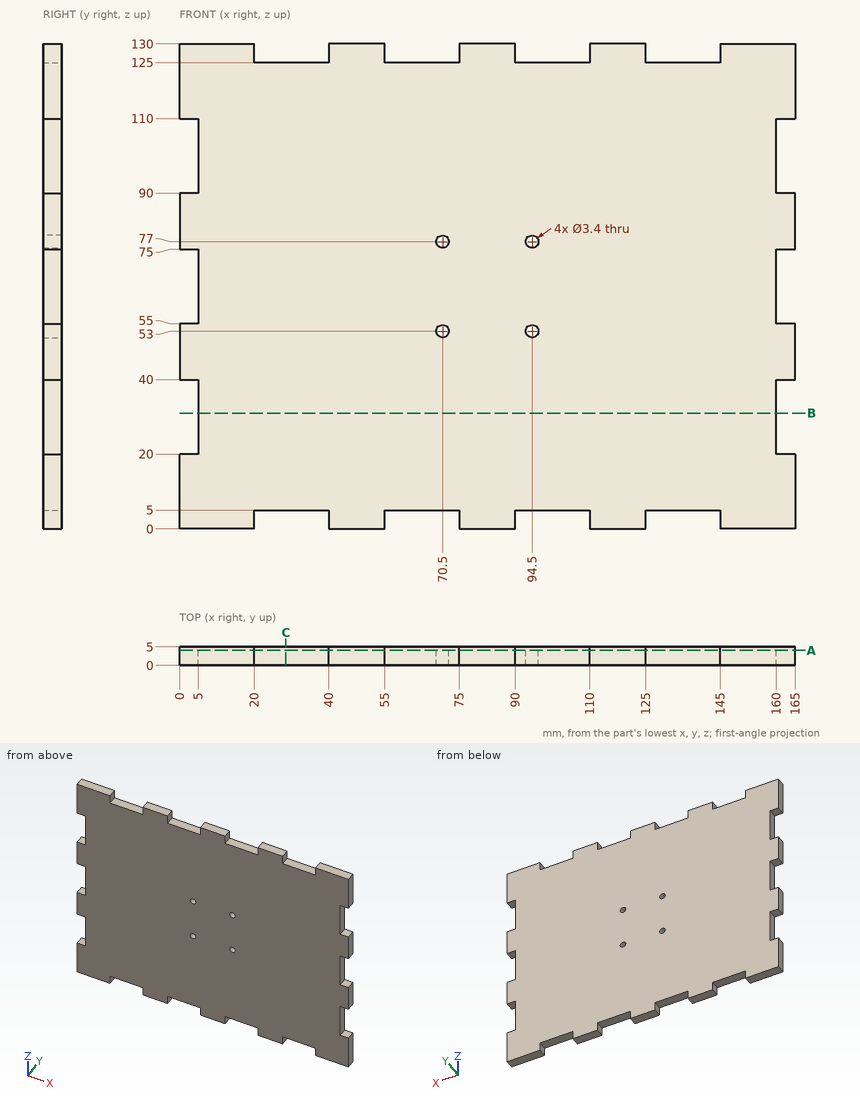
Check sheet for the drawn part. Datum: minimum x, y, z corner. Units: mm. Round coordinates to 2 decimals unless told otherwise and drop trailing zeros. Order: outer loops, then holes, each group sorted by start corner. A loop starts at its lowest first (then second) coordinate and runs counter-clockwise, first axis right, second up. Notation, with made-up numbers: (-37, 48.5) -> (-4, 48.5) arc R20 ccw to (-4, 55.5) -> close; hole circle Ø5 at (85.5, 57). An arc over 180 degrees is marked (long way). Put each result on its own line as item: value. Start each with the question number.
(1) Section check C-C (x = 28.5). Enter the section's corners in (y, z).
(2) Section check B-B (z = 31). Enter the section's corners in (x, y), then the cut area to 3 significant figures.
(3) Depth check by flat-ended pin: pin 1 Ø2.5 at (y, z) = (3, 2.5) entering from -X; pin 2 Ø2.5 at (y, z) = (3, 60.5) entering from -X; pin 3 Ø2.5 at (x, z) = (70.5, 77) entering from -Y; pin 4 Ø1.5 at (x, y) = (99, 2) entering from +Z. Enter the tip coordinate at first touch or a pass-through.
(4) Material ranges on line 1 along X through (y, z) = (3.55, 76.5); line 2 along Z through (x, y) = (69.5, 4.55); line 3 along X through (y, z) = (2.25, 58), recorded low to high.
(5) Section check A-A (y = 4.05). State how many separate pieces and enclosed holes the cut face has, then the cut area to 3 significant figures.
Completed:
1. outline: (0, 5) -> (5, 5) -> (5, 125) -> (0, 125) -> close
2. outline: (5, 0) -> (160, 0) -> (160, 5) -> (5, 5) -> close
2. area: 775 mm2
3. pin 1: stops at x = 0
3. pin 2: stops at x = 5
3. pin 3: passes through
3. pin 4: stops at z = 125
4. line 1: x = 0 to 68.88, 72.12 to 92.88, 96.12 to 165
4. line 2: z = 5 to 51.63, 54.37 to 75.63, 78.37 to 125
4. line 3: x = 5 to 160
5. separate pieces: 1
5. enclosed holes: 4
5. area: 20,000 mm2
